Check sheet for the modelled part. Datum: model origin and axes. Units: mm. Give positions to 0.01 mm unless a question says otherwise; leave off trailing zeros. Loops run counter-clockwise (first coordinate to the right, second up) from the corner with the lowest first, then second, coordinate; pieces in that order, holes last.
```python
from build123d import *

# Parameters (mm, degrees)
F0_W     = 25.4
F0_H     = 25.4
F1_DEPTH = 25.4
F2_SIZE  = 12.69999
F3_W     = 25.4
F3_H     = 12.7
F4_DEPTH = 25.4


# Not quite as in the source:
# - a fillet or chamfer is up to 0.001 mm smaller than in the source, because OpenCascade refuses the exact size


with BuildPart() as f1:
    # F0 (on Front) → F1 (new body)
    with BuildSketch(Plane.XZ):
        with Locations((-12459.5173980713, 4152.3379470825)):
            Rectangle(F0_W, F0_H)
    extrude(amount=F1_DEPTH)

    # F2 (size 12.7 in the source; OpenCascade refuses exactly that, so slightly less here)
    f2_edges = [f1.edges().sort_by_distance(p)[0] for p in [
        (-12446.817398, -25.4, 4152.337947),
        (-12459.517398, -25.4, 4139.637947),
        (-12472.217398, -25.4, 4152.337947),
        (-12459.517398, -25.4, 4165.037947),
    ]]
    chamfer(f2_edges, length=F2_SIZE)

    # F3 (on face) → F4 (cut)
    with BuildSketch(Plane(origin=(0, 0, 4139.6379470825), x_dir=(1, 0, 0), z_dir=(0, 0, -1))):
        with Locations((-12459.5173980713, 6.35)):
            Rectangle(F3_W, F3_H)
    extrude(amount=-F4_DEPTH, mode=Mode.SUBTRACT)


solid = f1.part
```
(1) Material ranges on line 1 (Z direction, x = -12466.75, y = -16.25); line 2 (Y direction, x = -12462.75, z = 4162.25); line 3 (X direction, y = -16.75, z = 4150.5), recorded low to high.
(2) Section check B-B on y = -21. Record the boundary of the cut face in (x, z).
(3) Section check A-A on x = -12450.5. Record the boundary of the cut face in (y, z), plus the area to 3 significant figures.
(4) Gauge pin test, flat ends, axial feed: pin 1 Ø1.5 at (y, z) = (-15.5, 4146) entering from +X; pin 2 Ø5 at (y, z) = (-22, 4149) entering from +X; pin 3 Ø2 at (x, y) = (-12466.5, -16.5) entering from -Z. Record the tip position at first contact, or that the pin passes through.
Computed values:
1. line 1: z = 4143.19 to 4161.49
1. line 2: y = -15.49 to -12.7
1. line 3: x = -12468.17 to -12450.87
2. outline: (-12463.92, 4147.94) - (-12455.12, 4147.94) - (-12455.12, 4156.74) - (-12463.92, 4156.74) - close
3. outline: (-16.38, 4143.32) - (-12.7, 4139.64) - (-12.7, 4165.04) - (-16.38, 4161.36) - close
3. area: 80.0 mm2
4. pin 1: stops at x = -12448.87
4. pin 2: stops at x = -12453.62
4. pin 3: stops at z = 4142.44
